Geometry check sheet. Reference: the model listing, model coordinates, mm. A direction names the side the tool comes from. Coordinates: 2 decimals unless noted, no trailing zeros. Write each loop counter-clockwise with the first axis right and the second up, starting at its lowest first coordinate (ties: lowest second). Pieces come first, ordered by that corner, then holes. Notation, with made-up numbers: M 14,62.25 L 19,62.25 A17 ccw 19,73.25 Z; hole C -21.5,82.5 d1. An arc over 180 degrees is marked long. Answer as a JSON object with one key per item and string values. Group by question number.
```python
from build123d import *

# Parameters (mm, degrees)
F0_R     = 1.35
F1_DEPTH = 9
F2_W     = 8.35
F2_H     = 19.2
F3_DEPTH = 8


with BuildPart() as f1:
    # F0 (on Top) → F1 (new body)
    with BuildSketch(Plane.XY):
        with BuildLine():
            Line((26.104286, 19.725), (-26.104286, 19.725))
            ThreePointArc((-26.104286, 19.725), (-30.815254, 20.815254), (-29.725, 16.104286))
            Line((-29.725, 16.104286), (-29.725, -16.104286))
            ThreePointArc((-29.725, -16.104286), (-30.815254, -20.815254), (-26.104286, -19.725))
            Line((-26.104286, -19.725), (26.104286, -19.725))
            ThreePointArc((26.104286, -19.725), (30.815254, -20.815254), (29.725, -16.104286))
            Line((29.725, -16.104286), (29.725, 16.104286))
            ThreePointArc((29.725, 16.104286), (30.815254, 20.815254), (26.104286, 19.725))
        make_face()
        with Locations((-28.8, -18.8)):
            Circle(F0_R, mode=Mode.SUBTRACT)
        with Locations((28.8, -18.8)):
            Circle(F0_R, mode=Mode.SUBTRACT)
        with Locations((-28.8, 18.8)):
            Circle(F0_R, mode=Mode.SUBTRACT)
        with Locations((28.8, 18.8)):
            Circle(F0_R, mode=Mode.SUBTRACT)
    extrude(amount=F1_DEPTH)

    # F2 (on face) → F3 (cut)
    with BuildSketch(Plane(origin=(0, 0, 0), x_dir=(1, 0, 0), z_dir=(0, 0, -1))):
        with Locations((-21.525, 0)):
            Rectangle(F2_W, F2_H)
    extrude(amount=-F3_DEPTH, mode=Mode.SUBTRACT)


solid = f1.part
```
1) Set-up check for faces 4 (the flat face through (29.725, 0, 4)), 5 (the flat face through (-25.7, 0, 4)), 6 (the flat face through (-29.725, 0, 4)), 7 (the flat face through (0, 19.725, 4)): record each of +Z, -Z, +X, -X, +Y, -Y from which the full face is reachable in a straight line by a thin tool's end or side.
2) Section check C-C (y = 18.8). Record the cut outline in (x, z), then the cut area to 3 significant figures.
3) Section check B-B (z = 1.5). Record the cut outline in (x, y) (3 decimals), then the cut area to 3 significant figures.
4) Section check D-D (y = -3.5). Record the cut outline in (x, z) (3 decimals), then the cut area to 3 significant figures.
5) Material ranges on probe 1 along Y at (x, z) = (-28.8, 6.75); probe 2 along X at (y, z) = (-8, 5.5) (3 decimals); probe 3 along X at (y, z) = (20, 6.25), recorded low to high. Write a range as [from, to].
6) Section check A-A (x = -28.8). Record the cut outline in (y, z).
7) Draft check along Y on faces 1 (the flat face through (0, 0, 0)), 2 (the cylindrical face through (27.45, -18.74, 4.44)), 3 (the flat face through (0, -19.725, 4)). Enter one of: +Y half, -Y half, draft (parallel to the pull), parting line (faces both ways), or undercut.
8) Go/stop test with flat-tipped pins: pin 1 Ø2.5 at (y, z) = (4.5, 6) entering from +X (3 decimals); pin 2 Ø1.5 at (x, z) = (8.5, 2) entering from +Y (3 decimals); pin 3 Ø4 at (y, z) = (-12.5, 4) entering from -X (3 decimals). Record where each tip stops, or that it passes through.
Entries:
{
 "1": {"face 4": "+Z, -Z, +X", "face 5": "-Z", "face 6": "+Z, -Z, -X", "face 7": "+Z, -Z, +Y"},
 "2": {"outline": "M -31.65,0 L -30.15,0 L -30.15,9 L -31.65,9 Z; M -27.45,0 L 27.45,0 L 27.45,9 L -27.45,9 Z; M 30.15,0 L 31.65,0 L 31.65,9 L 30.15,9 Z", "area": "521 mm^2"},
 "3": {"outline": "M -29.725,-16.104 A2.85 ccw long -26.104,-19.725 L 26.104,-19.725 A2.85 ccw long 29.725,-16.104 L 29.725,16.104 A2.85 ccw long 26.104,19.725 L -26.104,19.725 A2.85 ccw long -29.725,16.104 Z; hole C -28.8,-18.8 d2.7; hole C -28.8,18.8 d2.7; hole M -25.7,-9.6 L -17.35,-9.6 L -17.35,9.6 L -25.7,9.6 Z; hole C 28.8,-18.8 d2.7; hole C 28.8,18.8 d2.7", "area": "2,210 mm^2"},
 "4": {"outline": "M -29.725,0 L -25.7,0 L -25.7,8 L -17.35,8 L -17.35,0 L 29.725,0 L 29.725,9 L -29.725,9 Z", "area": "468 mm^2"},
 "5": {"probe 1": "[-21.65, -20.15], [-17.45, 17.45], [20.15, 21.65]", "probe 2": "[-29.725, -25.7], [-17.35, 29.725]", "probe 3": "[-31.39, -29.42], [-28.18, -26.21], [26.21, 28.18], [29.42, 31.39]"},
 "6": {"outline": "M -21.65,0 L -20.15,0 L -20.15,9 L -21.65,9 Z; M -17.45,0 L 17.45,0 L 17.45,9 L -17.45,9 Z; M 20.15,0 L 21.65,0 L 21.65,9 L 20.15,9 Z"},
 "7": {"face 1": "draft", "face 2": "undercut", "face 3": "-Y half"},
 "8": {"pin 1": "x = 29.725", "pin 2": "y = 19.725", "pin 3": "x = -29.725"}
}
